from build123d import *

# Parameters (mm, degrees)
SKETCH_2_W             = 20
SKETCH_2_H             = 6
EXTRUDE_379_DEPTH      = 5
SKETCH_3_R             = 4
CUT_EXTRUDE_526_DEPTH  = 16.362291496
SKETCH_4_R             = 5.25
CUT_EXTRUDE_602_DEPTH  = 2.25
SKETCH_5_R             = 1.25
CUT_EXTRUDE_755_DEPTH  = 13.68857754
CHAMFER_2_SIZE         = 1
SKETCH_6_R             = 2.3
CUT_EXTRUDE_1018_DEPTH = 1.5


with BuildPart() as part:
    # Эскиз2 → Extrude 379 (new, symmetric)
    with BuildSketch(Plane.XY):
        with Locations((0, 3)):
            Rectangle(SKETCH_2_W, SKETCH_2_H)
    extrude(amount=EXTRUDE_379_DEPTH, both=True)

    # Эскиз3 → Cut-Extrude 526 (cut, through all)
    with BuildSketch(Plane.XY.offset(5)):
        Circle(SKETCH_3_R)
    extrude(amount=-CUT_EXTRUDE_526_DEPTH, mode=Mode.SUBTRACT)

    # Эскиз4 → Cut-Extrude 602 (cut, symmetric)
    with BuildSketch(Plane.XY):
        Circle(SKETCH_4_R)
    extrude(amount=CUT_EXTRUDE_602_DEPTH, both=True, mode=Mode.SUBTRACT)

    # Эскиз5 → Cut-Extrude 755 (cut, through all)
    with BuildSketch(Plane(origin=(0, 6, 0), x_dir=(1, 0, 0), z_dir=(0, 1, 0))):
        with Locations(Location((-7, 0, 0), (0, 0, 270))):
            Circle(SKETCH_5_R)
        with Locations(Location((7, 0, 0), (0, 0, 270))):
            Circle(SKETCH_5_R)
    extrude(amount=-CUT_EXTRUDE_755_DEPTH, mode=Mode.SUBTRACT)

    # Фаска2
    chamfer_2_edges = [part.edges().sort_by_distance(p)[0] for p in [
        (0, 4, 5),
        (0, 4, -5),
    ]]
    chamfer(chamfer_2_edges, length=CHAMFER_2_SIZE)

    # Эскиз6 → Cut-Extrude 1018 (cut)
    with BuildSketch(Plane(origin=(0, 6, 0), x_dir=(1, 0, 0), z_dir=(0, 1, 0))):
        with Locations(Location((-7, 0, 0), (0, 0, 270))):
            Circle(SKETCH_6_R)
        with Locations(Location((7, 0, 0), (0, 0, 270))):
            Circle(SKETCH_6_R)
    extrude(amount=-CUT_EXTRUDE_1018_DEPTH, mode=Mode.SUBTRACT)


solid = part.part
The listing builds one solid part. Answer for the finished solid, in the listing's coordinates (mm). A direction names the side the tool comes from. Coordinates: 2 decimals unless noted, no trailing zeros. Loops run counter-clockwise (first coordinate to the right, second up) from the corner with the lowest first, then second, coordinate; pieces in that order, holes last.
1) Find section D-D on x = 0. Write down the section's boundary in (y, z).
2) Find section C-C on y = 5.45. Write down the section's boundary in (x, z).
3) Find section A-A on x = 7. Write down the section's boundary in (y, z), then the cut area to 4 significant figures.
4) A tool of negligible diameter and unlimited length cuts with its end or side. For faces 1 (the face through (-8, 4.5, 1)), 2 (the face through (0, 4, -3)), 3 (the face through (0.4, 4.2, 2.25)), from which of +Z, -Z, +X, -X, +Y, -Y can it reach the whole face along a straight path? Write none if from no direction.
5) Flat-ended cylindrical pins translate along their axes: pin 1 Ø3 at (x, z) = (5.5, -3.5) entering from -Y; pin 2 Ø3 at (x, z) = (7, 0) entering from +Y; pin 3 Ø2.5 at (x, y) = (2.5, 1.5) entering from +Z; pin 4 Ø2.5 at (x, y) = (0.5, 3) entering from -Z. Find the tip coordinate at first contact, or state that the pin passes through.
6) Find section B-B on z = 0. Write down the section's boundary in (x, y).
7) Find the intervals of material crossed by L1, parallel to X at y = 1.8, z = 0; L2, parallel to X at y = 1.5, z = 0; L3, parallel to Y at x = -6.25, z = 1.5, in increasing order.
8) Determine the mould class of faces 4 (the face through (-0.1, 5.7, 5)), 5 (the face through (7.691, 5.26, 2.194)), 6 (the face through (-0.1, 5.7, -5)), 7 (the face through (10, 3, 0)) for opening direction Z: pulls with the +Z half, pulls with the -Z half, needs draft (parallel to the pull), parting line crosses it, or undercut.
Values:
1. outline: (4, -4) - (5, -5) - (6, -5) - (6, 5) - (5, 5) - (4, 4) - (4, 2.25) - (5.25, 2.25) - (5.25, -2.25) - (4, -2.25) - close
2. outline: (-10, -5) - (10, -5) - (10, 5) - (-10, 5) - close; hole circle Ø4.6 at (-7, 0); hole circle Ø4.6 at (7, 0)
3. outline: (0, -5) - (6, -5) - (6, -2.3) - (4.5, -2.3) - (4.5, -1.25) - (0, -1.25) - close; (0, 1.25) - (4.5, 1.25) - (4.5, 2.3) - (6, 2.3) - (6, 5) - (0, 5) - close
3. area: 41.85 mm2
4. face 1: +Y
4. face 2: +Z, -Z, -Y
4. face 3: -Y
5. pin 1: stops at y = 0
5. pin 2: stops at y = 4.5
5. pin 3: stops at z = 4.17
5. pin 4: stops at z = -4.29
6. outline: (-10, 0) - (-8.25, 0) - (-8.25, 4.5) - (-9.3, 4.5) - (-9.3, 6) - (-10, 6) - close; (-5.75, 0) - (-5.25, 0) arc R5.25 cw to (5.25, 0) - (5.75, 0) - (5.75, 4.5) - (4.7, 4.5) - (4.7, 6) - (-4.7, 6) - (-4.7, 4.5) - (-5.75, 4.5) - close; (8.25, 0) - (10, 0) - (10, 6) - (9.3, 6) - (9.3, 4.5) - (8.25, 4.5) - close
7. L1: x = -10 to -8.25, -5.75 to -4.93, 4.93 to 5.75, 8.25 to 10
7. L2: x = -10 to -8.25, -5.75 to -5.03, 5.03 to 5.75, 8.25 to 10
7. L3: y = 0 to 4.5
8. face 4: pulls with the +Z half
8. face 5: undercut
8. face 6: pulls with the -Z half
8. face 7: needs draft
